Answer from the drawing. Dimensions are ordinates in mm from the lowest x, y and z of the part. A direction names the side the tool comes from. Give positions to 0.01 mm unless a question says otherwise; leave off trailing zeros. Write each loop counter-clockwise with the first axis right and the second up, starting at its lowest first coordinate (ties: lowest second). Pieces come first, ordered by that corner, then holes.
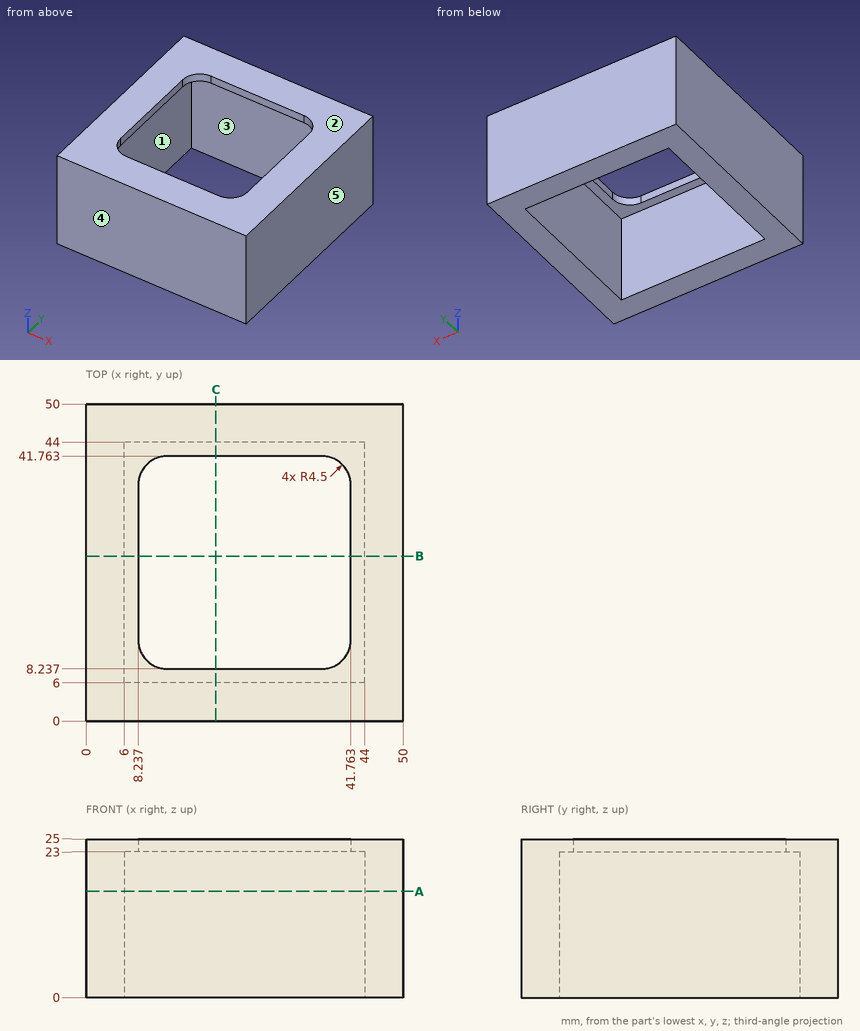
Item 1: Which of the six approach directions +Z, -Z, +X, -X, +Y, -Y give full straight-line access (tool end or side, diameter ignored) to the marked faces 1 and 2?
Conclusion:
face 1: -Z
face 2: +Z, +X, -X, +Y, -Y
Item 2: A cutting plane is placed at A-A, the plane z = 16.75. Give the vertices of the cut face in (x, y).
Conclusion:
outline: (0, 0) - (50, 0) - (50, 50) - (0, 50) - close; hole (6, 6) - (44, 6) - (44, 44) - (6, 44) - close
Item 3: A cutting plane is placed at B-B, the plane y = 26. Give the vertices of the cut face in (x, z), plus the area to 3 significant figures.
Conclusion:
outline: (0, 0) - (6, 0) - (6, 23) - (8.24, 23) - (8.24, 25) - (0, 25) - close; (41.76, 23) - (44, 23) - (44, 0) - (50, 0) - (50, 25) - (41.76, 25) - close
area: 309 mm2
Item 4: Determine the mould class of the marked faces 3, 4 and 5 for opening direction Y: pulls with the +Y half, pulls with the -Y half, needs draft (parallel to the pull), parting line crosses it, or undercut.
Conclusion:
face 3: undercut
face 4: pulls with the -Y half
face 5: needs draft
Item 5: Consider probe 1 along X at (y, z) = (32, 16). Determine where the line is inside the solid, lowest interval first.
Conclusion:
probe 1: x = 0 to 6, 44 to 50
